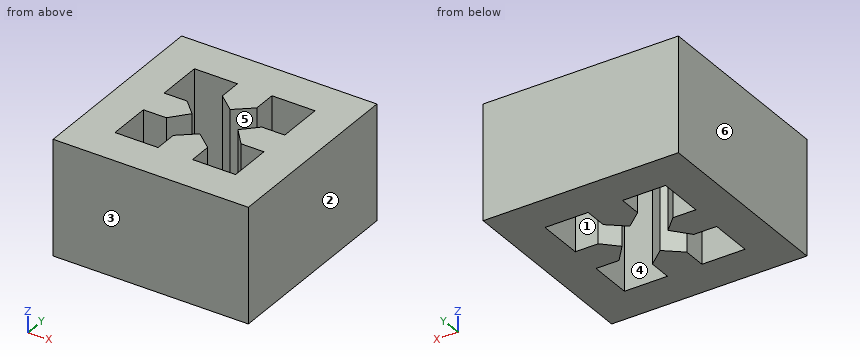
from build123d import *

# Parameters (mm, degrees)
SKETCH_W     = 34
SKETCH_H     = 34
PAD_DEPTH    = 20
POCKET_DEPTH = 20


with BuildPart() as part:
    # Sketch → Pad (new body)
    with BuildSketch(Plane.XY):
        with Locations((17, 17)):
            Rectangle(SKETCH_W, SKETCH_H)
    extrude(amount=PAD_DEPTH)

    # Sketch001 (on Face6 of Pad) → Pocket (cut)
    with BuildSketch(Plane.XY.offset(20)):
        Polygon((6.5, 27.5), (14, 27.5), (14, 23.5), (17, 21), (20, 23.5), (20, 27.5), (27.5, 27.5), (27.5, 19.5), (23.5, 19.5), (21, 17), (23.5, 14), (27.5, 14), (27.5, 6.5), (20, 6.5), (20, 10.5), (17, 13), (14, 10.5), (14, 6.5), (6.5, 6.5), (6.5, 14), (10.5, 14), (13, 17), (10.5, 19.5), (6.5, 19.5), align=None)
    extrude(amount=-POCKET_DEPTH, mode=Mode.SUBTRACT)


solid = part.part
Model file for the job. Use its own axes, mm. Face numbers are marked on the shaded views. A direction names the side the tool comes from. Give positions to 0.01 mm unless a question says otherwise; leave off trailing zeros. Write each loop counter-clockwise with the first axis right and the second up, starting at its lowest first coordinate (ties: lowest second). Pieces come first, ordered by that corner, then holes. Notation, with made-up numbers: (-13.5, -7.5) - (39.5, -7.5) arc R20 ccw to (39.5, 20.5) - close; hole circle Ø5 at (-2.75, 11.25). An arc over 180 degrees is marked (long way). Answer as CSV lines item,"result".
1. Band-saw the part on B-B (y = 10). Write the cut outline in (x, z).
Responses:
outline,"(0, 0) - (6.5, 0) - (6.5, 20) - (0, 20) - close; (14, 0) - (20, 0) - (20, 20) - (14, 20) - close; (27.5, 0) - (34, 0) - (34, 20) - (27.5, 20) - close"
2. 3-axis set-ups, long thin cutter, end or side, ignore diameter. For the marked faces 1 and 2: which of +Z, -Z, +X, -X, +Y, -Y reach the whole face in a straight line?
Responses:
face 1,"+Z, -Z"
face 2,"+Z, -Z, +X, +Y, -Y"
3. Band-saw the part on A-A (x = 13.5). Write the cut outline in (y, z), and give its area (3 significant figures).
Responses:
outline,"(0, 0) - (6.5, 0) - (6.5, 20) - (0, 20) - close; (27.5, 0) - (34, 0) - (34, 20) - (27.5, 20) - close"
area,"260 mm2"
4. Band-saw the part on D-D (x = 25). Write the cut outline in (y, z), and give its area (3 significant figures).
Responses:
outline,"(0, 0) - (6.5, 0) - (6.5, 20) - (0, 20) - close; (14, 0) - (19.5, 0) - (19.5, 20) - (14, 20) - close; (27.5, 0) - (34, 0) - (34, 20) - (27.5, 20) - close"
area,"370 mm2"
5. Drill centre lines: L1, parallel to X at y = 7, z = 10.25; L2, parallel to Y at x = 25, z = 10.75; L3, parallel to Y at x = 11, z = 7.5. Where is each one in solid material? Low to high. Write a range as [from, to].
Responses:
L1,"x = [0, 6.5], [14, 20], [27.5, 34]"
L2,"y = [0, 6.5], [14, 19.5], [27.5, 34]"
L3,"y = [0, 6.5], [14.6, 19], [27.5, 34]"
6. Two-plate mould, pull along Y, no slides. Class the marked faces 3, 4, 5 and 6: +Y half, -Y half, draft (parallel to the pull), parting line (faces both ways), or undercut.
Responses:
face 3,"-Y half"
face 4,"undercut"
face 5,"undercut"
face 6,"draft"
7. Band-saw the part on C-C (z = 5.5). Write the cut outline in (x, y).
Responses:
outline,"(0, 0) - (34, 0) - (34, 34) - (0, 34) - close; hole (6.5, 6.5) - (14, 6.5) - (14, 10.5) - (17, 13) - (20, 10.5) - (20, 6.5) - (27.5, 6.5) - (27.5, 14) - (23.5, 14) - (21, 17) - (23.5, 19.5) - (27.5, 19.5) - (27.5, 27.5) - (20, 27.5) - (20, 23.5) - (17, 21) - (14, 23.5) - (14, 27.5) - (6.5, 27.5) - (6.5, 19.5) - (10.5, 19.5) - (13, 17) - (10.5, 14) - (6.5, 14) - close"
